Job drawing, mm, ordinate dimensions from the low corner. One solid piece. A direction names the side the tool comes from. Give positions to 0.01 mm unless a question says otherwise; leave off trailing zeros. Write each loop counter-clockwise with the first axis right and the second up, starting at its lowest first coordinate (ties: lowest second). Pieces come first, ordered by that corner, then holes. Notation, with made-up numbers: (11.5, 15) -> (25.5, 15) arc R25 ccw to (25.5, 52) -> close; hole circle Ø7 at (32.5, 24.25). An arc over 180 degrees is marked (long way). One line per question, with ' | ' between items. Start each with the question number.
(1) Tool access for the marked faces 1 and 2: list every direction of +Z, -Z, +X, -X, +Y, -Y with a clear straight run to the whole face (end or side of a thin tool).
(2) Band-saw the part on A-A, the plane y = 28. Give the cut face in (x, z) (1 decimal).
(3) Band-saw the part on C-C, the plane x = 40. Give the cut face in (y, z) (1 decimal).
(4) Drill centre lines: probe 1 along Y at (x, z) = (37.5, 17) (1 decimal); probe 2 along X at (y, z) = (29.5, 17.5) (1 decimal); probe 3 along Y at (x, z) = (24.5, 3) (1 decimal). Where is each one in solid material? Low to high. Write a range as from..to.
(5) Pin check, flat tips, straight feed: P1, Ø10, axis at y = 47.5, z = 34.5, coming from the -X side (1 decimal); P2, Ø10, axis at x = 51.5, z = 21.5, coming from the -Y side; P3, Ø4, axis at x = 41, z = 14.5, coming from the -Y side. Stop position of each tip, or through.
(6) Band-saw the part on D-D, the plane y = 8. Give the cut face in (x, z), and give its area (3 significant figures).
(7) Pull direction Y, two halves, no side cores. Call the marked faces 3, 4 and 5: released by +Y, released by -Y, zero draft, split by the parting line, or undercut.
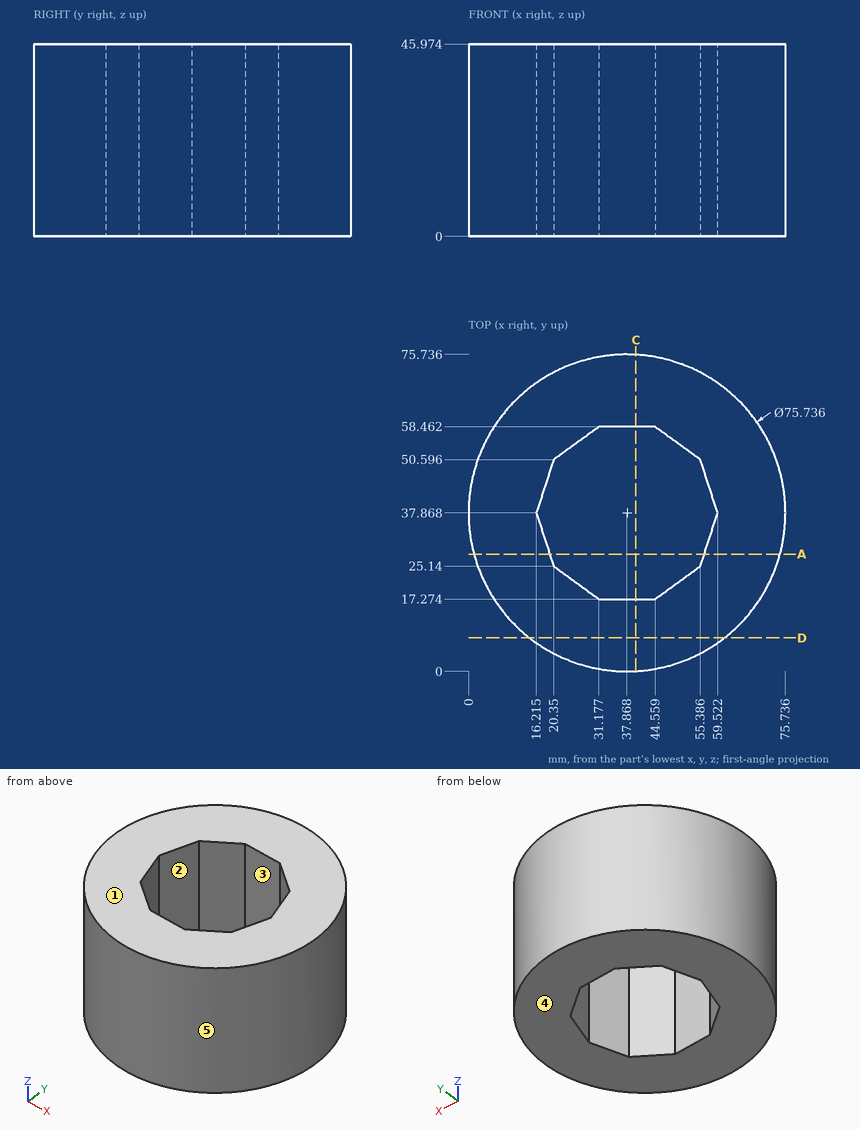
Results:
1) face 1: +Z, +X, -X, +Y, -Y | face 2: +Z, -Z
2) outline: (1.3, 0) -> (19.4, 0) -> (19.4, 46) -> (1.3, 46) -> close; (56.3, 0) -> (74.4, 0) -> (74.4, 46) -> (56.3, 46) -> close
3) outline: (0.1, 0) -> (17.3, 0) -> (17.3, 46) -> (0.1, 46) -> close; (58.5, 0) -> (75.7, 0) -> (75.7, 46) -> (58.5, 46) -> close
4) probe 1: y = 0..17.3, 58.5..75.7 | probe 2: x = 0.9..18.9, 56.8..74.8 | probe 3: y = 2.4..22.1, 53.6..73.3
5) P1: stops at x = 0.3 | P2: stops at y = 1 | P3: stops at y = 0.02
6) outline: (14.59, 0) -> (61.15, 0) -> (61.15, 45.97) -> (14.59, 45.97) -> close | area: 2,140 mm²
7) face 3: undercut | face 4: zero draft | face 5: split by the parting line
